The drawing under review shows one solid part. Ordinate dimensions are in mm from its lowest x, y, z. Give positions to 0.01 mm unless a question says otherwise; leave off trailing zeros. Write each loop counter-clockwise with the first axis right and the second up, starting at its lowest first coordinate (ties: lowest second). Pieces come first, ordered by that corner, then holes. Notation, with made-up numbers: (77.25, -5) -> (106.25, -5) arc R10 cw to (106.25, -1) -> close; hole circle Ø11 at (-25.5, 21.5). An arc over 180 degrees is marked (long way). Write item = value, one per line.
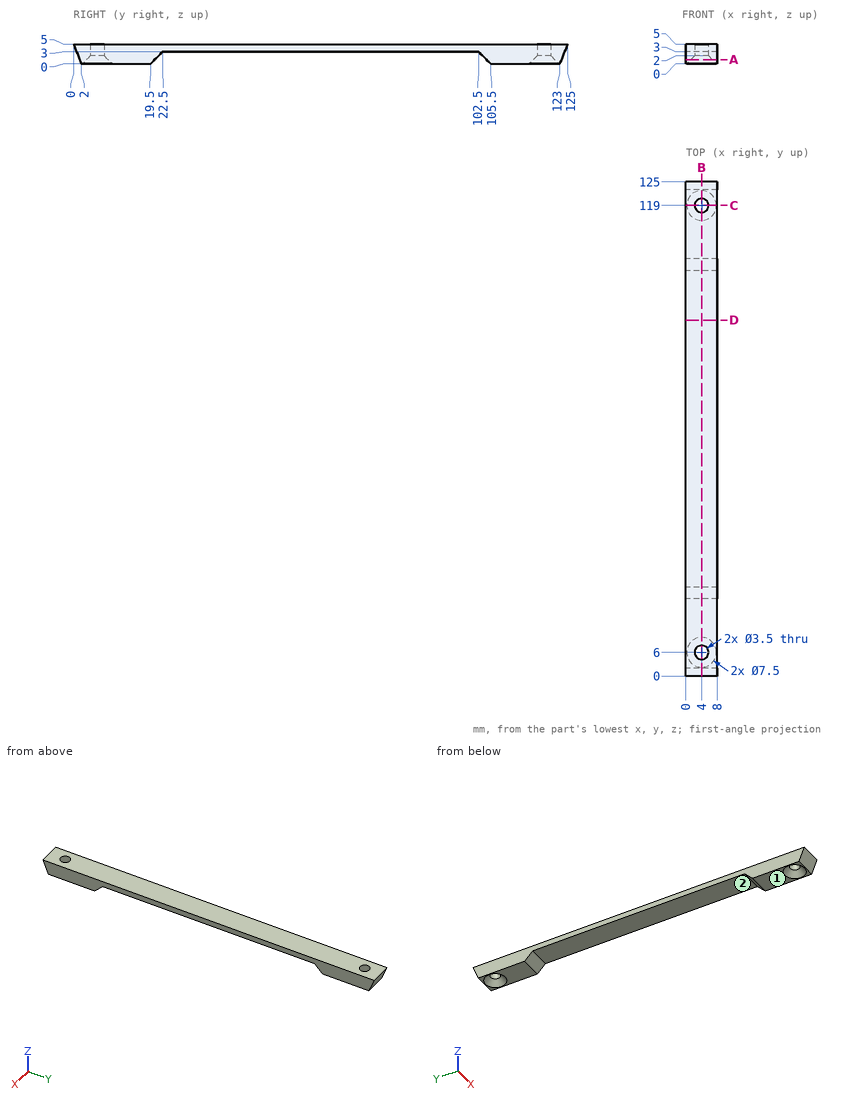
(1) Take a section at B-B (x = 4). Write out the cut boundary in (y, z).
Answers below:
outline = (0, 5) -> (2, 0) -> (2.25, 0) -> (4.25, 2) -> (4.25, 5) -> close; (7.75, 2) -> (9.75, 0) -> (19.5, 0) -> (22.5, 3) -> (102.5, 3) -> (105.5, 0) -> (115.25, 0) -> (117.25, 2) -> (117.25, 5) -> (7.75, 5) -> close; (120.75, 2) -> (122.75, 0) -> (123, 0) -> (125, 5) -> (120.75, 5) -> close
(2) To check wall thickness, follow probe 1 along Y at (x, z) = (5, 0.45); probe 2 along Y at (x, z) = (1, 0.35); probe 3 along X at (y, z) = (119, 3.1). State the ranges of each line that lie inside material, in increasing order.
Answers below:
probe_1 = 1.82 to 2.86, 9.14 to 19.95, 105.05 to 115.86, 122.14 to 123.18
probe_2 = 1.86 to 4.4, 7.6 to 19.85, 105.15 to 117.4, 120.6 to 123.14
probe_3 = 0 to 2.25, 5.75 to 8
(3) Take a section at D-D (y = 90). Write out the cut boundary in (x, z), plus the area to 3 significant figures.
Answers below:
outline = (0, 3) -> (8, 3) -> (8, 5) -> (0, 5) -> close
area = 16.0 mm^2
(4) For pin 1 (1 mm diameter, centred on x = 2.5, z = 2.5, fed in from -Y); pin 2 (3 mm diameter, centred on x = 5, z = 2, fed in from +Y); pin 3 (3 mm diameter, centred on x = 6.5, z = 2, fed in from -Y), all flat-tipped, find the tip position at first contact; note any pin that passes through.
Answers below:
pin_1 = 0.8
pin_2 = 124.4
pin_3 = 0.6
(5) The part is to be moulded in two halves that separate along Y. For the marked faces 1 and 2, say which applies: released by +Y, released by -Y, zero draft, split by the parting line, or undercut.
Answers below:
face_1 = zero draft
face_2 = undercut
(6) Take a section at A-A (z = 1.05). Write out the cut boundary in (x, y), plus the area to 3 significant figures.
Answers below:
outline = (0, 1.58) -> (8, 1.58) -> (8, 20.55) -> (0, 20.55) -> close; (0, 104.45) -> (8, 104.45) -> (8, 123.42) -> (0, 123.42) -> close; hole circle Ø5.4 at (4, 6); hole circle Ø5.4 at (4, 119)
area = 258 mm^2
(7) Take a section at C-C (y = 119). Write out the cut boundary in (x, z).
Answers below:
outline = (0, 0) -> (0.25, 0) -> (2.25, 2) -> (2.25, 5) -> (0, 5) -> close; (5.75, 2) -> (7.75, 0) -> (8, 0) -> (8, 5) -> (5.75, 5) -> close
